Could you check a few things on this model? Use its own coordinates, in mm. Face numbers are marked on the shaded views. Round coordinates to 2 decimals unless told otherwise and drop trailing zeros. Write each loop counter-clockwise with the first axis right and the second up, starting at its lowest first coordinate (ties: lowest second). Pieces come first, ordered by that corner, then holes. Notation, with made-up numbers: (83, 13) -> (121, 13) arc R24 cw to (121, 37) -> close; hole circle Ø1 at (-11.5, 22.5). An arc over 180 degrees is marked (long way). Answer in a Markdown table with one row per item.
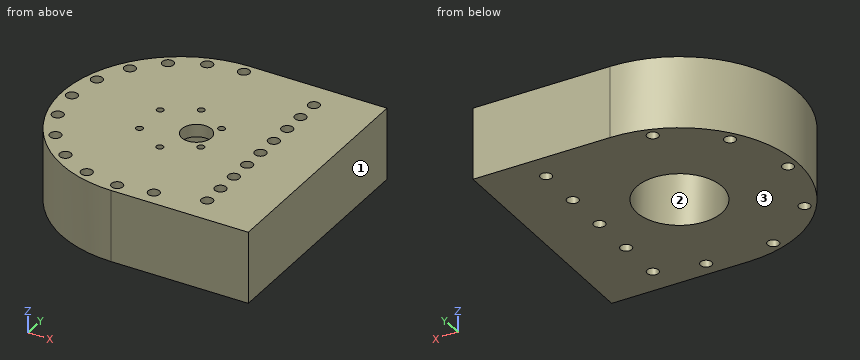
from build123d import *

# Parameters (mm, degrees)
CROQUIS1_R              = 18.725
SALIENTE_EXTRUIR1_DEPTH = 26
CROQUIS2_R              = 6.5
CROQUIS2_R_2            = 1.5
SALIENTE_EXTRUIR2_DEPTH = 5.5
CROQUIS3_R              = 2.5
CORTAR_EXTRUIR1_DEPTH   = 86.418089419
CROQUIS4_R              = 2.5
CORTAR_EXTRUIR2_DEPTH   = 20


with BuildPart() as part:
    # Croquis1 → Saliente-Extruir1 (new body)
    with BuildSketch(Plane.XY):
        with BuildLine():
            Line((0, 52), (60, 52))
            Line((60, 52), (60, -52))
            Line((60, -52), (0, -52))
            ThreePointArc((0, -52), (-52, 0), (0, 52))
        make_face()
        with Locations(Location((0, 0, 0), (0, 0, 180))):
            Circle(CROQUIS1_R, mode=Mode.SUBTRACT)
    extrude(amount=SALIENTE_EXTRUIR1_DEPTH)

    # Croquis2 → Saliente-Extruir2 (add)
    with BuildSketch(Plane.XY.offset(26)):
        with BuildLine():
            Line((0, -52), (60, -52))
            Line((60, -52), (60, 52))
            Line((60, 52), (0, 52))
            ThreePointArc((0, 52), (-52, 0), (0, -52))
        make_face()
        with Locations((7, 0)):
            Circle(CROQUIS2_R, mode=Mode.SUBTRACT)
        with Locations((13.423393759, -7.75)):
            Circle(CROQUIS2_R_2, mode=Mode.SUBTRACT)
        with Locations((13.423393759, 7.75)):
            Circle(CROQUIS2_R_2, mode=Mode.SUBTRACT)
        with Locations((0, 15.5)):
            Circle(CROQUIS2_R_2, mode=Mode.SUBTRACT)
        with Locations((0, -15.5)):
            Circle(CROQUIS2_R_2, mode=Mode.SUBTRACT)
        with Locations((-13.423393759, -7.75)):
            Circle(CROQUIS2_R_2, mode=Mode.SUBTRACT)
        with Locations((-13.423393759, 7.75)):
            Circle(CROQUIS2_R_2, mode=Mode.SUBTRACT)
    extrude(amount=SALIENTE_EXTRUIR2_DEPTH)

    # Croquis3 → Cortar-Extruir1 (cut, through all)
    with BuildSketch(Plane.XY.offset(31.5)):
        with Locations((35, 0)):
            Circle(CROQUIS3_R)
        with Locations((35, 20)):
            Circle(CROQUIS3_R)
        with Locations((35, 40)):
            Circle(CROQUIS3_R)
        with Locations(Location((35, -40, 0), (0, 0, 180))):
            Circle(CROQUIS3_R)
        with Locations(Location((35, -20, 0), (0, 0, 180))):
            Circle(CROQUIS3_R)
        with Locations((-14.678307233, 45.175184524)):
            Circle(CROQUIS3_R)
        with Locations((-38.428307233, 27.919799484)):
            Circle(CROQUIS3_R)
        with Locations((-47.5, 0)):
            Circle(CROQUIS3_R)
        with Locations((-38.428307233, -27.919799484)):
            Circle(CROQUIS3_R)
        with Locations((-14.678307233, -45.175184524)):
            Circle(CROQUIS3_R)
        with Locations((14.678307233, -45.175184524)):
            Circle(CROQUIS3_R)
    extrude(amount=-CORTAR_EXTRUIR1_DEPTH, mode=Mode.SUBTRACT)

    # Croquis4 → Cortar-Extruir2 (cut)
    with BuildSketch(Plane.XY.offset(31.5)):
        with Locations((0, 47.5)):
            Circle(CROQUIS4_R)
        with Locations((-27.919799484, 38.428307233)):
            Circle(CROQUIS4_R)
        with Locations((-45.175184524, 14.678307233)):
            Circle(CROQUIS4_R)
        with Locations((-45.175184524, -14.678307233)):
            Circle(CROQUIS4_R)
        with Locations((-27.919799484, -38.428307233)):
            Circle(CROQUIS4_R)
        with Locations((0, -47.5)):
            Circle(CROQUIS4_R)
        with Locations((35, 30)):
            Circle(CROQUIS4_R)
        with Locations((35, 10)):
            Circle(CROQUIS4_R)
        with Locations((35, -10)):
            Circle(CROQUIS4_R)
        with Locations((35, -30)):
            Circle(CROQUIS4_R)
    extrude(amount=-CORTAR_EXTRUIR2_DEPTH, mode=Mode.SUBTRACT)


solid = part.part
1) For pin 1 (1.5 mm diameter, centred on x = -17, y = 29.5, fed in from -Z); pin 2 (1 mm diameter, centred on x = -38.5, z = 23.5, fed in from +Y); pin 3 (6 mm diameter, centred on x = -24.5, z = 18, fed in from +Y); pin 4 (6 mm diameter, centred on y = 22.5, z = 10.5, fed in from -X), each with a flat end and sliding along its axis, tell me the tip position at first contact or that it passes through.
Findings:
| item | result |
|---|---|
| pin 1 | stops at z = 0 |
| pin 2 | stops at y = 35.5 |
| pin 3 | stops at y = 47.35 |
| pin 4 | stops at x = -48.21 |
2) Please list where these lines run through material, in increasing order: line 1 (Y direction, x = 0, z = 23) (3 decimals); line 2 (Y direction, x = 16.5, z = 25.5); line 3 (X direction, y = 39, z = 29.5).
Findings:
| item | result |
|---|---|
| line 1 | y = -52 to -50, -45 to -18.725, 18.725 to 45, 50 to 52 |
| line 2 | y = -52 to -46.89, -43.46 to -8.85, 8.85 to 52 |
| line 3 | x = -34.39 to -30.35, -25.49 to 32.71, 37.29 to 60 |
3) Imagine slicing it at B-B, the plane x = -37.5. Please give me the cut outline in (y, z).
Findings:
| item | result |
|---|---|
| outline | (-36.02, 0) -> (-30.24, 0) -> (-30.24, 31.5) -> (-36.02, 31.5) -> close; (-25.6, 0) -> (25.6, 0) -> (25.6, 31.5) -> (-25.6, 31.5) -> close; (30.24, 0) -> (36.02, 0) -> (36.02, 31.5) -> (30.24, 31.5) -> close |
4) Imagine slicing it at C-C, the plane z = 2. Count the separate pieces of the cut face and the enclosed holes in it, plus the area to 3 significant figures.
Findings:
| item | result |
|---|---|
| separate pieces | 1 |
| enclosed holes | 12 |
| area | 9,170 mm^2 |
5) Thinking about a two-plate mould opening in X: for the marked faces 1, 2 and 3, which applies, +X half, -X half, draft (parallel to the pull), parting line (faces both ways), or undercut?
Findings:
| item | result |
|---|---|
| face 1 | +X half |
| face 2 | undercut |
| face 3 | draft |
6) Imagine slicing it at A-A, the plane y = -20. Please give me the cut outline in (x, z), plus the area to 3 significant figures.
Findings:
| item | result |
|---|---|
| outline | (-48, 0) -> (32.5, 0) -> (32.5, 31.5) -> (-48, 31.5) -> close; (37.5, 0) -> (60, 0) -> (60, 31.5) -> (37.5, 31.5) -> close |
| area | 3,240 mm^2 |
